```python
from build123d import *

# Parameters (mm, degrees)
BOSS_EXTRU_2_DEPTH      = 40
ESQUISSE2_W             = 55
ESQUISSE2_H             = 12
BOSS_EXTRU_3_DEPTH      = 40
BOSS_EXTRU_4_DEPTH      = 12
ESQUISSE4_R             = 7.5
ENL_V_MAT_EXTRU_1_DEPTH = 96.655632349


with BuildPart() as part:
    # Esquisse1 → Boss.-Extru.2 (new body)
    with BuildSketch(Plane(origin=(0, 0, 0), x_dir=(1, 0, 0), z_dir=(0, 1, 0))):
        Polygon((0, 0), (0, 23), (55, 23), (55, 0), (40, 0), (40, 18), (15, 18), (15, 0), align=None)
    extrude(amount=BOSS_EXTRU_2_DEPTH)

    # Esquisse2 → Boss.-Extru.3 (add)
    with BuildSketch(Plane(origin=(0, 0, 0), x_dir=(1, 0, 0), z_dir=(0, 1, 0))):
        with Locations((27.5, 29)):
            Rectangle(ESQUISSE2_W, ESQUISSE2_H)
    extrude(amount=BOSS_EXTRU_3_DEPTH)

    # Esquisse3 → Boss.-Extru.4 (add)
    with BuildSketch(Plane(origin=(0, 0, -35), x_dir=(-1, 0, 0), z_dir=(0, 0, -1))):
        with BuildLine():
            Line((-55, 40), (-55, 62.307284183))
            ThreePointArc((-55, 62.307284183), (-27.5, 70), (0, 62.307284183))
            Line((0, 62.307284183), (0, 40))
            Line((0, 40), (-55, 40))
        make_face()
    extrude(amount=-BOSS_EXTRU_4_DEPTH)

    # Esquisse4 → Enlèv. mat.-Extru.1 (cut, through all)
    with BuildSketch(Plane(origin=(0, 0, -35), x_dir=(-1, 0, 0), z_dir=(0, 0, -1))):
        with Locations((-27.5, 17)):
            Circle(ESQUISSE4_R)
    extrude(amount=-ENL_V_MAT_EXTRU_1_DEPTH, mode=Mode.SUBTRACT)


solid = part.part
```
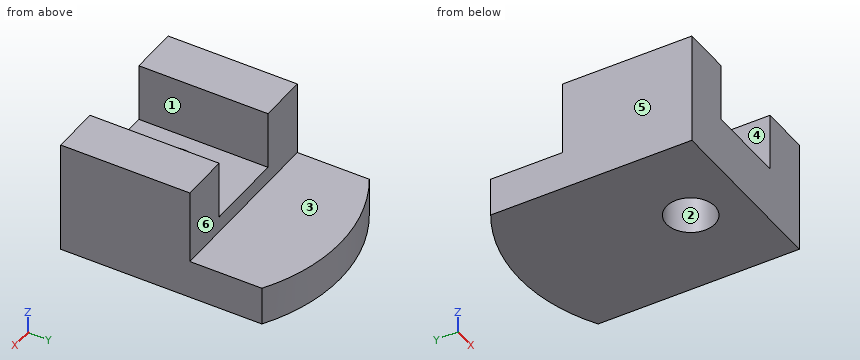
Geometry check sheet. Reference: the model listing, model coordinates, mm. Face numbers are marked on the shaded views. A direction names the side the tool comes from. Round coordinates to 2 decimals unless told otherwise and drop trailing zeros. Order: outer loops, then holes, each group sorted by start corner. A loop starts at its lowest first (then second) coordinate and runs counter-clockwise, first axis right, second up. Notation, with made-up numbers: (20.5, 75.25) - (78.5, 75.25) arc R33 ccw to (78.5, 103.25) - close; hole circle Ø11 at (27, 17). An arc over 180 degrees is marked (long way). Use a Markdown table: item, result. Add a question column.
(1) Sectioned sample at A-A, the plane y = 17. Enter the section's corners in (x, z), and give its area (3 significant figures).
(2) Sectioned sample at D-D, the plane x = 6. Enter the section's corners in (y, z).
(3) Sectioned sample at C-C, the plane y = 25.5. Enter the section's corners in (x, z).
(4) Material ranges on line 1 along Y through (x, z) = (27, -22); line 2 along X through (y, z) = (19, -5.5); line 3 along Y through (x, z) = (27, -26), recorded low to high. Write a range as [from, to].
(5) Depth check by flat-ended pin: pin 1 (12 mm diameter, centred on x = 26.5, z = -6, fed in from +Y); pin 2 (18.5 mm diameter, centred on x = 38.5, z = -7.5, fed in from +Y). Enter the tip coordinate at first touch or a pass-through.
(6) Release check for a two-part mould opening along X. For the marked faces 4, 5 and 6 record: pulls with the +X half, pulls with the -X half, needs draft (parallel to the pull), parting line crosses it, or undercut.
(7) Sectioned sample at B-B, the plane x = 27.5. Enter the section's corners in (y, z).
(8) Tool access check on the marked faces 1, 2 and 3. Record the directions out of +Z, -Z, +X, -X, +Y, -Y that give a thin tool (end or side, any length) a straight path to the whole face; none if there is none.
Answers below:
| question | item | result |
|---|---|---|
| 1 | outline | (0, -35) - (20, -35) - (20, -18) - (15, -18) - (15, 0) - (0, 0) - close; (35, -35) - (55, -35) - (55, 0) - (40, 0) - (40, -18) - (35, -18) - close |
| 1 | area | 1,220 mm² |
| 2 | outline | (0, -35) - (65.44, -35) - (65.44, -23) - (40, -23) - (40, 0) - (0, 0) - close |
| 3 | outline | (0, -35) - (55, -35) - (55, 0) - (40, 0) - (40, -18) - (15, -18) - (15, 0) - (0, 0) - close |
| 4 | line 1 | [0, 9.52], [24.48, 40] |
| 4 | line 2 | [0, 15], [40, 55] |
| 4 | line 3 | [0, 9.52], [24.48, 70] |
| 5 | pin 1 | through |
| 5 | pin 2 | y = 40 |
| 6 | face 4 | undercut |
| 6 | face 5 | pulls with the -X half |
| 6 | face 6 | needs draft |
| 7 | outline | (0, -35) - (9.5, -35) - (9.5, -18) - (0, -18) - close; (24.5, -35) - (70, -35) - (70, -23) - (40, -23) - (40, -18) - (24.5, -18) - close |
| 8 | face 1 | +Z, +Y, -Y |
| 8 | face 2 | +Z, -Z |
| 8 | face 3 | +Z, +X, -X, +Y |
